```python
from build123d import *

# Parameters (mm, degrees)
SKETCH_1_W          = 25
SKETCH_1_H          = 50
EXTRUDE_1_DEPTH     = 521.512
CUT_EXTRUDE_1_DEPTH = 521.51
CUT_EXTRUDE_2_DEPTH = 521.51


with BuildPart() as part:
    # Эскиз1 → Бобышка-Вытянуть1 (new body)
    with BuildSketch(Plane(origin=(0, 0, 0), x_dir=(1, 0, 0), z_dir=(0, 1, 0))):
        Rectangle(SKETCH_1_W, SKETCH_1_H)
    extrude(amount=EXTRUDE_1_DEPTH)

    # Эскиз2 → Вырез-Вытянуть1 (cut)
    with BuildSketch(Plane(origin=(12.5, 0, 0), x_dir=(0, 0, -1), z_dir=(1, 0, 0))):
        Polygon((-25, 521.512), (0, 521.512), (-25, 496.512), align=None)
        Polygon((25, 0), (25, 25.90361446), (-25, 0), align=None)
    extrude(amount=-CUT_EXTRUDE_1_DEPTH, mode=Mode.SUBTRACT)

    # Эскиз3 → Вырез-Вытянуть2 (cut)
    with BuildSketch(Plane(origin=(12.5, 0, 0), x_dir=(0, 0, -1), z_dir=(1, 0, 0))):
        Polygon((0, 521.512), (25, 496.512), (25, 521.512), align=None)
    extrude(amount=-CUT_EXTRUDE_2_DEPTH, mode=Mode.SUBTRACT)


solid = part.part
```
Design review of the part built by this model. Coordinates are the model's own, in mm. Give positions to 0.01 mm unless a question says otherwise; leave off trailing zeros. Write each loop counter-clockwise with the first axis right and the second up, starting at its lowest first coordinate (ties: lowest second). Pieces come first, ordered by that corner, then holes.
(1) Clearance check with flat-ended pins moving along their axes: pin 1 Ø1 at (x, z) = (2, -19.5) entering from +Y; pin 2 Ø3 at (x, z) = (-3, -10) entering from -Y; pin 3 Ø1 at (x, z) = (1, 0) entering from -Y. State where each tip first meets the part, or that it passes through.
Checked values:
pin 1: stops at y = 502.51
pin 2: stops at y = 17.36
pin 3: stops at y = 12.69
(2) Add section C-C (z = -17.5). Give the boundary of the cut face in (x, y), and give its area (3 significant figures).
Checked values:
outline: (-12.5, 22.02) - (12.5, 22.02) - (12.5, 504.01) - (-12.5, 504.01) - close
area: 12,000 mm2
(3) Wall thickness on line 1 along Y through (x, z) = (-9.5, 21.5); line 2 along Y through (x, z) = (-2.5, 21): over which ranges is each line inside the solid? List them lowest first.
Checked values:
line 1: y = 1.81 to 500.01
line 2: y = 2.07 to 500.51
(4) Add section B-B (z = 16.5). Give the boundary of the cut face in (x, y).
Checked values:
outline: (-12.5, 4.4) - (12.5, 4.4) - (12.5, 505.01) - (-12.5, 505.01) - close
(5) Add section A-A (x = 5.25). Give the boundary of the cut face in (y, z), and give its area (3 significant figures).
Checked values:
outline: (0, 25) - (25.9, -25) - (496.51, -25) - (521.51, 0) - (496.51, 25) - close
area: 24,800 mm2
